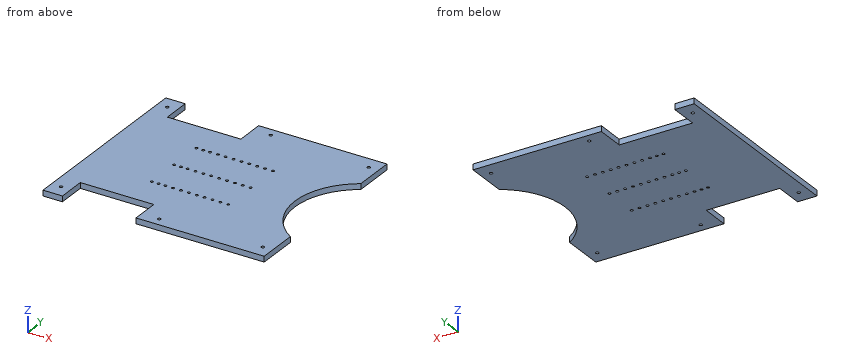
```python
from build123d import *

# Parameters (mm, degrees)
SKETCH1_R           = 1.7525
SKETCH1_R_2         = 1.5
BOSS_EXTRUDE1_DEPTH = 6.35


with BuildPart() as part:
    # Sketch1 → Boss-Extrude1 (new body)
    with BuildSketch(Plane.XY):
        with BuildLine():
            Line((119.609790965, 110), (97.609790965, 110))
            Line((97.609790965, 110), (14.609790965, 110))
            Line((14.609790965, 110), (-25.390209035, 110))
            Line((-25.390209035, 110), (-25.390209035, 78))
            Line((-25.390209035, 78), (-108.390209035, 78))
            Line((-108.390209035, 78), (-108.390209035, 110))
            Line((-108.390209035, 110), (-130.390209035, 110))
            Line((-130.390209035, 110), (-130.390209035, -110))
            Line((-130.390209035, -110), (-108.390209035, -110))
            Line((-108.390209035, -110), (-108.390209035, -78))
            Line((-108.390209035, -78), (-25.390209035, -78))
            Line((-25.390209035, -78), (-25.390209035, -110))
            Line((-25.390209035, -110), (14.609790965, -110))
            Line((14.609790965, -110), (97.609790965, -110))
            Line((97.609790965, -110), (119.609790965, -110))
            Line((119.609790965, -110), (119.609790965, -63.2))
            ThreePointArc((119.609790965, -63.2), (84.992460515, 0), (119.609790965, 63.2))
            Line((119.609790965, 63.2), (119.609790965, 110))
        make_face()
        with Locations((-119.390209035, 95)):
            Circle(SKETCH1_R, mode=Mode.SUBTRACT)
        with Locations(Location((108.609790965, 95, 0), (0, 0, 180))):
            Circle(SKETCH1_R, mode=Mode.SUBTRACT)
        with Locations((-5.390209035, 100)):
            Circle(SKETCH1_R, mode=Mode.SUBTRACT)
        with Locations(Location((-5.390209035, -100, 0), (0, 0, 180))):
            Circle(SKETCH1_R, mode=Mode.SUBTRACT)
        with Locations((108.609790965, -95)):
            Circle(SKETCH1_R, mode=Mode.SUBTRACT)
        with Locations(Location((-119.390209035, -95, 0), (0, 0, 180))):
            Circle(SKETCH1_R, mode=Mode.SUBTRACT)
        with Locations((-36.311771099, 40)):
            Circle(SKETCH1_R_2, mode=Mode.SUBTRACT)
        with Locations((-36.311771099, 0)):
            Circle(SKETCH1_R_2, mode=Mode.SUBTRACT)
        with Locations(Location((-36.311771099, -40, 0), (0, 0, 180))):
            Circle(SKETCH1_R_2, mode=Mode.SUBTRACT)
        with Locations(Location((-27.421771099, -40, 0), (0, 0, 180))):
            Circle(SKETCH1_R_2, mode=Mode.SUBTRACT)
        with Locations((-27.421771099, 0)):
            Circle(SKETCH1_R_2, mode=Mode.SUBTRACT)
        with Locations((-27.421771099, 40)):
            Circle(SKETCH1_R_2, mode=Mode.SUBTRACT)
        with Locations(Location((-18.531771099, -40, 0), (0, 0, 180))):
            Circle(SKETCH1_R_2, mode=Mode.SUBTRACT)
        with Locations((-18.531771099, 0)):
            Circle(SKETCH1_R_2, mode=Mode.SUBTRACT)
        with Locations((-18.531771099, 40)):
            Circle(SKETCH1_R_2, mode=Mode.SUBTRACT)
        with Locations(Location((-9.641771099, -40, 0), (0, 0, 180))):
            Circle(SKETCH1_R_2, mode=Mode.SUBTRACT)
        with Locations((-9.641771099, 0)):
            Circle(SKETCH1_R_2, mode=Mode.SUBTRACT)
        with Locations((-9.641771099, 40)):
            Circle(SKETCH1_R_2, mode=Mode.SUBTRACT)
        with Locations(Location((-0.751771099, -40, 0), (0, 0, 180))):
            Circle(SKETCH1_R_2, mode=Mode.SUBTRACT)
        with Locations((-0.751771099, 0)):
            Circle(SKETCH1_R_2, mode=Mode.SUBTRACT)
        with Locations((-0.751771099, 40)):
            Circle(SKETCH1_R_2, mode=Mode.SUBTRACT)
        with Locations(Location((8.138228901, -40, 0), (0, 0, 180))):
            Circle(SKETCH1_R_2, mode=Mode.SUBTRACT)
        with Locations((8.138228901, 0)):
            Circle(SKETCH1_R_2, mode=Mode.SUBTRACT)
        with Locations((8.138228901, 40)):
            Circle(SKETCH1_R_2, mode=Mode.SUBTRACT)
        with Locations(Location((17.028228901, -40, 0), (0, 0, 180))):
            Circle(SKETCH1_R_2, mode=Mode.SUBTRACT)
        with Locations((17.028228901, 0)):
            Circle(SKETCH1_R_2, mode=Mode.SUBTRACT)
        with Locations((17.028228901, 40)):
            Circle(SKETCH1_R_2, mode=Mode.SUBTRACT)
        with Locations(Location((25.918228901, -40, 0), (0, 0, 180))):
            Circle(SKETCH1_R_2, mode=Mode.SUBTRACT)
        with Locations((25.918228901, 0)):
            Circle(SKETCH1_R_2, mode=Mode.SUBTRACT)
        with Locations((25.918228901, 40)):
            Circle(SKETCH1_R_2, mode=Mode.SUBTRACT)
        with Locations(Location((34.808228901, -40, 0), (0, 0, 180))):
            Circle(SKETCH1_R_2, mode=Mode.SUBTRACT)
        with Locations((34.808228901, 0)):
            Circle(SKETCH1_R_2, mode=Mode.SUBTRACT)
        with Locations((34.808228901, 40)):
            Circle(SKETCH1_R_2, mode=Mode.SUBTRACT)
        with Locations((-43.931771099, 0)):
            Circle(SKETCH1_R_2, mode=Mode.SUBTRACT)
        with Locations(Location((-43.931771099, -40, 0), (0, 0, 180))):
            Circle(SKETCH1_R_2, mode=Mode.SUBTRACT)
        with Locations((-43.931771099, 40)):
            Circle(SKETCH1_R_2, mode=Mode.SUBTRACT)
        with Locations((-51.551771099, 0)):
            Circle(SKETCH1_R_2, mode=Mode.SUBTRACT)
        with Locations(Location((-51.551771099, -40, 0), (0, 0, 180))):
            Circle(SKETCH1_R_2, mode=Mode.SUBTRACT)
        with Locations((-51.551771099, 40)):
            Circle(SKETCH1_R_2, mode=Mode.SUBTRACT)
    extrude(amount=BOSS_EXTRUDE1_DEPTH)


solid = part.part
```
The listing builds one solid part. Answer for the finished solid, in the listing's coordinates (mm). Round coordinates to 2 decimals unless told otherwise and drop trailing zeros. Loops run counter-clockwise (first coordinate to the right, second up) from the corner with the lowest first, then second, coordinate; pieces in that order, holes last. Notation, with made-up numbers: (15.25, 39) - (45.25, 39) arc R32 ccw to (45.25, 70) - close; hole circle Ø6 at (77.5, 4.25). An arc over 180 degrees is marked (long way). Return JSON: item names as keys, results as strings. Group by question number.
1. The part is cut by section B-B on x = -32. Determine the outline of the cut face in (y, z), then the cut area to 3 significant figures.
2. The part is cut by section A-A on z = 4.75. State how many separate pieces and enclosed holes the cut face has, then the cut area to 3 significant figures.
3. The part is cut by section C-C on y = 5. Determine the outline of the cut face in (x, z), then the cut area to 3 significant figures.
4. Consider probe 1 along Y at (x, z) = (25.5, 4.5); probe 2 along X at (y, z) = (95, 3.5); probe 3 along Y at (x, z) = (97.5, 3.25). Determine where each line is inside the solid, lowest interval first.
Resolved:
{
 "1": {"outline": "(-78, 0) - (78, 0) - (78, 6.35) - (-78, 6.35) - close", "area": "991 mm²"},
 "2": {"separate pieces": "1", "enclosed holes": "39", "area": "46,300 mm²"},
 "3": {"outline": "(-130.39, 0) - (85.16, 0) - (85.16, 6.35) - (-130.39, 6.35) - close", "area": "1,370 mm²"},
 "4": {"probe 1": "y = -110 to -41.44, -38.56 to -1.44, 1.44 to 38.56, 41.44 to 110", "probe 2": "x = -130.39 to -121.14, -117.64 to -108.39, -25.39 to 106.86, 110.36 to 119.61", "probe 3": "y = -110 to -41.47, 41.47 to 110"}
}
